Design review of the part built by this model. Coordinates are the model's own, in mm. Coordinates: 2 decimals unless noted, no trailing zeros. Write each loop counter-clockwise with the first axis right and the second up, starting at its lowest first coordinate (ties: lowest second). Pieces come first, ordered by that corner, then holes. Notation, with made-up numbers: M 27,-26 L 52,-26 A20 ccw 52,3 Z; hole C -36,52.25 d2. An arc over 180 degrees is marked long. Write item = value, one per line.
```python
from build123d import *

# Parameters (mm, degrees)
SKETCH1_W          = 25.4
SKETCH1_H          = 177.8
BASE_EXTRUDE_DEPTH = 25.4
SKETCH2_R          = 7.62
CUT_EXTRUDE1_DEPTH = 78.74
FILLET1_R          = 2.54


with BuildPart() as part:
    # Sketch1 → Base-Extrude (new body)
    with BuildSketch(Plane.XY):
        with Locations((-7.849662618, -19.144264507)):
            Rectangle(SKETCH1_W, SKETCH1_H)
    extrude(amount=BASE_EXTRUDE_DEPTH)

    # Sketch2 → Cut-Extrude1 (cut)
    with BuildSketch(Plane.XY.offset(25.4)):
        with Locations((-7.849662618, -95.344264507)):
            Circle(SKETCH2_R)
        with Locations((-7.849662618, 57.055735493)):
            Circle(SKETCH2_R)
    extrude(amount=-CUT_EXTRUDE1_DEPTH, mode=Mode.SUBTRACT)

    # Fillet1
    fillet1_edges = [part.edges().sort_by_distance(p)[0] for p in [
        (-20.549662618, 69.755735493, 12.7),
        (4.850337382, 69.755735493, 12.7),
        (-7.849662618, 69.755735493, 0),
        (-7.849662618, 69.755735493, 25.4),
        (-20.549662618, -108.044264507, 12.7),
        (4.850337382, -108.044264507, 12.7),
        (-7.849662618, -108.044264507, 0),
        (-7.849662618, -108.044264507, 25.4),
    ]]
    fillet(fillet1_edges, radius=FILLET1_R)


solid = part.part
```
Q1. Consider section A-A, the plane x = -11. State the section outline as (y, z) points.
Check result:
outline = M -108.04,2.54 A2.54 ccw -105.5,0 L -102.28,0 L -102.28,25.4 L -105.5,25.4 A2.54 ccw -108.04,22.86 Z; M -88.41,0 L 50.12,0 L 50.12,25.4 L -88.41,25.4 Z; M 63.99,0 L 67.22,0 A2.54 ccw 69.76,2.54 L 69.76,22.86 A2.54 ccw 67.22,25.4 L 63.99,25.4 Z
Q2. Consider section B-B, the plane z = 17.5. State the section outline as (x, y) points, and give its area (3 significant figures).
Check result:
outline = M -20.55,-105.5 A2.54 ccw -18.01,-108.04 L 2.31,-108.04 A2.54 ccw 4.85,-105.5 L 4.85,67.22 A2.54 ccw 2.31,69.76 L -18.01,69.76 A2.54 ccw -20.55,67.22 Z; hole C -7.85,-95.34 d15.24; hole C -7.85,57.06 d15.24
area = 4,150 mm²
Q3. The part is to be moulded in two halves that separate along X. For faces 1 (the flat face through (-8, -108.044, 13)), 2 (the cylindrical face through (-8.84, 64.61, 12.88)), 3 (the flat face through (4.85, -20, 13)), say which applies: +X half, -X half, draft (parallel to the pull), parting line (faces both ways), or undercut.
Check result:
face_1 = draft
face_2 = undercut
face_3 = +X half
Q4. Wall thickness on line 1 (Y direction, x = -7.5, z = 23.25); line 2 (Y direction, x = -11, z = 22); line 3 (Y direction, x = 0.75, z = 23.25): over which ranges is each line inside the solid? List them lowest first.
Check result:
line_1 = -108.01 to -102.96, -87.73 to 49.44, 64.67 to 69.73
line_2 = -108.04 to -102.28, -88.41 to 50.12, 63.99 to 69.76
line_3 = -108.01 to 69.73
